Design review of the part built by this model. Coordinates are the model's own, in mm. Coordinates: 2 decimals unless noted, no trailing zeros. Write each loop counter-clockwise with the first axis right and the second up, starting at its lowest first coordinate (ties: lowest second). Pieces come first, ordered by that corner, then holes. Notation, with made-up numbers: (77, -40) - (97, -40) arc R22 cw to (97, -14) - close; hole circle Ø8 at (-1.75, -27). An arc over 180 degrees is marked (long way). Use a Markdown table: item, result.
from build123d import *

# Parameters (mm, degrees)
F1_DEPTH = 12.7
F3_DEPTH = 25.4


with BuildPart() as f1:
    # F0 (on Front) → F1 (new body)
    with BuildSketch(Plane.XZ):
        with BuildLine():
            Line((0, 38.1), (0, 0))
            Line((0, 0), (215.9, 0))
            ThreePointArc((215.9, 0), (242.840768, 11.159232), (254, 38.1))
            ThreePointArc((254, 38.1), (242.840768, 65.040768), (215.9, 76.2))
            Line((215.9, 76.2), (0, 76.2))
            Line((0, 76.2), (0, 38.1))
        make_face()
        with BuildLine():
            ThreePointArc((228.6, 38.1), (215.9, 25.4), (203.2, 38.1))
            ThreePointArc((203.2, 38.1), (215.9, 50.8), (228.6, 38.1))
        make_face(mode=Mode.SUBTRACT)
    extrude(amount=F1_DEPTH)

    # F2 (on face) → F3 (cut)
    with BuildSketch(Plane.XZ.offset(12.7)):
        with BuildLine():
            Line((194.8942, 20.3708), (194.8942, 22.7838))
            ThreePointArc((194.8942, 22.7838), (193.187951, 18.664551), (197.3072, 20.3708))
            Line((197.3072, 20.3708), (194.8942, 20.3708))
        make_face()
        with BuildLine():
            ThreePointArc((197.3072, 20.3708), (196.600449, 22.077049), (194.8942, 22.7838))
            Line((194.8942, 22.7838), (194.8942, 20.3708))
            Line((194.8942, 20.3708), (197.3072, 20.3708))
        make_face()
        with BuildLine():
            Line((236.9058, 55.8292), (234.4928, 55.8292))
            ThreePointArc((234.4928, 55.8292), (235.199551, 54.122951), (236.9058, 53.4162))
            Line((236.9058, 53.4162), (236.9058, 55.8292))
        make_face()
        with BuildLine():
            ThreePointArc((239.3188, 55.8292), (236.9058, 58.2422), (234.4928, 55.8292))
            Line((234.4928, 55.8292), (236.9058, 55.8292))
            Line((236.9058, 55.8292), (236.9058, 53.4162))
            ThreePointArc((236.9058, 53.4162), (238.612049, 54.122951), (239.3188, 55.8292))
        make_face()
    extrude(amount=-F3_DEPTH, mode=Mode.SUBTRACT)


solid = f1.part
(1) Draft analysis for pull direction X (two halves, no side actions). For faces 1 (the flat face through (0, -6, 39)), 2 (the cylindrical face through (228.588, -6.261, 38.658)), 3 (the flat face through (106, -6, 0)), state which applies: +X half, -X half, draft (parallel to the pull), parting line (faces both ways), or undercut.
Determined:
| item | result |
|---|---|
| face 1 | -X half |
| face 2 | undercut |
| face 3 | draft |
(2) For pin 1 (1.5 mm diameter, centred on y = -10, z = 23.5, fed in from +X), flat-tipped, find the tip position at first contact; note if it passes through.
Determined:
| item | result |
|---|---|
| pin 1 | x = 251.39 |
(3) For L1, parallel to Z at x = 215.9, y = -7.5; L2, parallel to X at y = -8.5, z = 43.5; L3, parallel to X at y = -5, z = 55, list the stretches that pass through material, from the lowest coordinate up. Write a range as from..to.
Determined:
| item | result |
|---|---|
| L1 | 0..25.4, 50.8..76.2 |
| L2 | 0..204.41, 227.39..253.62 |
| L3 | 0..234.64, 239.17..250.05 |
(4) Take a section at A-A on y = -8.5. Write out the cut boundary in (x, z), and give its area (3 significant figures).
Determined:
| item | result |
|---|---|
| outline | (0, 0) - (215.9, 0) arc R38.1 ccw to (254, 38.1) arc R38.1 ccw to (215.9, 76.2) - (0, 76.2) - close; hole (194.89, 22.78) arc R2.41 ccw (long way) to (197.31, 20.37) arc R2.41 ccw to start; hole circle Ø25.4 at (215.9, 38.1); hole (234.49, 55.83) arc R2.41 ccw to (236.91, 53.42) arc R2.41 ccw to (239.32, 55.83) arc R2.41 ccw to start |
| area | 18,200 mm2 |
(5) Take a section at C-C on z = 10.5. Write out the cut boundary in (x, y) (3 decimals).
Determined:
| item | result |
|---|---|
| outline | (0, -12.7) - (242.165, -12.7) - (242.165, 0) - (0, 0) - close |
(6) Take a section at B-B on z = 45. Write out the cut boundary in (x, y), and give its area (3 significant figures).
Determined:
| item | result |
|---|---|
| outline | (0, -12.7) - (205.24, -12.7) - (205.24, 0) - (0, 0) - close; (226.56, -12.7) - (253.37, -12.7) - (253.37, 0) - (226.56, 0) - close |
| area | 2,950 mm2 |
